Part model, mm, in its own coordinate system. Face numbers are marked on the shaded views. Round coordinates to 2 decimals unless told otherwise and drop trailing zeros. Loops run counter-clockwise (first coordinate to the right, second up) from the corner with the lowest first, then second, coordinate; pieces in that order, holes last. Notation, with made-up numbers: M 87.25,49 L 129.25,49 A31 cw 129.25,86 Z; hole C 89.5,5 d9. An arc over 180 degrees is marked long. Put each result on its own line as item: value. Start each with the question number.
1) Slice it at B-B on x = 7. Give the cut face in (y, z), then the cut area to 3 significant figures.
2) Probe line 1 along X through (y, z) = (30.1, 1.1); line 2 along Y through (x, z) = (30.1, 8); line 3 along X through (y, z) = (-28, 6). List the from-to ranges inside material, lowest first.
3) Slice it at C-C on x = -19. Give the cut face in (y, z), then the cut area to 3 significant figures.
4) Pull direction Y, two halves, no side cores. Call the marked faces 1 and 2: +Y half, -Y half, draft (parallel to the pull), parting line (faces both ways), or undercut.
5) Drop flat-ended pins along their axis: pin 1 Ø7 at (x, y) = (28.5, 28.5) entering from +Z; pin 2 Ø10 at (x, y) = (-26, -5) entering from +Z; pin 3 Ø2 at (x, z) = (7, 9.5) entering from -Y. Give the stop position or say it passes through.
6) Slice it at A-A on z = 9.5. State how many separate pieces and enclosed holes the cut face has, then the cut area to 3 significant figures.
```python
from build123d import *

# Parameters (mm, degrees)
SKETCH1_W            = 80.2
SKETCH1_H            = 80.2
BOSS_EXTRUDE1_DEPTH  = 4.5
M5_CLEARANCE_HOLE1_D = 5.3
FILLET1_R            = 10
SKETCH3_W            = 4
SKETCH3_H            = 18
BOSS_EXTRUDE2_DEPTH  = 10
CUT_EXTRUDE1_REACH   = 67.031
SKETCH5_R            = 2.4
CUT_EXTRUDE2_REACH   = 67.031
SKETCH6_R            = 1.75
FILLET2_R            = 2
FILLET3_R            = 4
BOSS_EXTRUDE3_START  = 6
SKETCH7_R            = 4.25
SKETCH7_R_2          = 2.65
BOSS_EXTRUDE3_DEPTH  = 6
FILLET5_R            = 1


with BuildPart() as part:
    # Sketch1 → Boss-Extrude1 (new body)
    with BuildSketch(Plane.XY):
        Rectangle(SKETCH1_W, SKETCH1_H)
    extrude(amount=BOSS_EXTRUDE1_DEPTH)

    # M5 Clearance Hole1 (through all)
    with Locations(Plane(origin=(30.1, 30.1, 0), x_dir=(-1, 0, 0), z_dir=(0, 0, -1))):
        with Locations((0, 0), (60.2, 0), (60.2, -60.2), (0, -60.2)):
            Hole(M5_CLEARANCE_HOLE1_D / 2)

    # Fillet1
    fillet1_edges = [part.edges().sort_by_distance(p)[0] for p in [
        (-40.1, -40.1, 2.25),
        (-40.1, 40.1, 2.25),
        (40.1, 40.1, 2.25),
        (40.1, -40.1, 2.25),
    ]]
    fillet(fillet1_edges, radius=FILLET1_R)

    # Sketch3 → Boss-Extrude2 (add)
    with BuildSketch(Plane.XY.offset(4.5)):
        with Locations((-7, 31.1)):
            Rectangle(SKETCH3_W, SKETCH3_H)
        with Locations((7, 31.1)):
            Rectangle(SKETCH3_W, SKETCH3_H)
    extrude(amount=BOSS_EXTRUDE2_DEPTH)

    # Sketch5 → Cut-Extrude1 (cut, up to next)
    with BuildSketch(Plane(origin=(9, 0, 0), x_dir=(0, 0, -1), z_dir=(1, 0, 0)), mode=Mode.PRIVATE) as cut_extrude1_sk1:
        with Locations(Location((-9.5, 36.1, 0), (0, 0, 90))):
            Circle(SKETCH5_R)
    cut_extrude1_tool1 = extrude(cut_extrude1_sk1.sketch, amount=-CUT_EXTRUDE1_REACH, mode=Mode.PRIVATE) & part.part
    # Sketch5 → Cut-Extrude1 (cut, up to next)
    with BuildSketch(Plane(origin=(9, 0, 0), x_dir=(0, 0, -1), z_dir=(1, 0, 0)), mode=Mode.PRIVATE) as cut_extrude1_sk2:
        with Locations(Location((-9.5, 26.1, 0), (0, 0, 90))):
            Circle(SKETCH5_R)
    cut_extrude1_tool2 = extrude(cut_extrude1_sk2.sketch, amount=-CUT_EXTRUDE1_REACH, mode=Mode.PRIVATE) & part.part
    add(cut_extrude1_tool1.solids().sort_by_distance((9, 36.1, 9.5))[0], mode=Mode.SUBTRACT)
    add(cut_extrude1_tool2.solids().sort_by_distance((9, 26.1, 9.5))[0], mode=Mode.SUBTRACT)

    # Sketch6 → Cut-Extrude2 (cut, up to next)
    with BuildSketch(Plane.ZY.offset(9), mode=Mode.PRIVATE) as cut_extrude2_sk1:
        with Locations((9.5, 36.1)):
            Circle(SKETCH6_R)
    cut_extrude2_tool1 = extrude(cut_extrude2_sk1.sketch, amount=-CUT_EXTRUDE2_REACH, mode=Mode.PRIVATE) & part.part
    # Sketch6 → Cut-Extrude2 (cut, up to next)
    with BuildSketch(Plane.ZY.offset(9), mode=Mode.PRIVATE) as cut_extrude2_sk2:
        with Locations((9.5, 26.1)):
            Circle(SKETCH6_R)
    cut_extrude2_tool2 = extrude(cut_extrude2_sk2.sketch, amount=-CUT_EXTRUDE2_REACH, mode=Mode.PRIVATE) & part.part
    add(cut_extrude2_tool1.solids().sort_by_distance((-9, 36.1, 9.5))[0], mode=Mode.SUBTRACT)
    add(cut_extrude2_tool2.solids().sort_by_distance((-9, 26.1, 9.5))[0], mode=Mode.SUBTRACT)

    # Fillet2
    fillet2_edges = [part.edges().sort_by_distance(p)[0] for p in [
        (-7, 22.1, 14.5),
        (-7, 40.1, 14.5),
        (7, 40.1, 14.5),
        (7, 22.1, 14.5),
    ]]
    fillet(fillet2_edges, radius=FILLET2_R)

    # Fillet3
    fillet3_edges = [part.edges().sort_by_distance(p)[0] for p in [
        (-7, 22.1, 4.5),
        (7, 22.1, 4.5),
    ]]
    fillet(fillet3_edges, radius=FILLET3_R)

    # Sketch7 → Boss-Extrude3 (add)
    # profile 1 of 4: a face of its own
    with BuildSketch(Plane.XY.offset(4.5).offset(BOSS_EXTRUDE3_START)):
        with Locations((-30.1, 30.1)):
            Circle(SKETCH7_R)
        with Locations(Location((-30.1, 30.1, 0), (0, 0, 180))):
            Circle(SKETCH7_R_2, mode=Mode.SUBTRACT)
    # profile 2 of 4: a face of its own
    with BuildSketch(Plane.XY.offset(4.5).offset(BOSS_EXTRUDE3_START)):
        with Locations((30.1, 30.1)):
            Circle(SKETCH7_R)
        with Locations(Location((30.1, 30.1, 0), (0, 0, 180))):
            Circle(SKETCH7_R_2, mode=Mode.SUBTRACT)
    # profile 3 of 4: a face of its own
    with BuildSketch(Plane.XY.offset(4.5).offset(BOSS_EXTRUDE3_START)):
        with Locations((30.1, -30.1)):
            Circle(SKETCH7_R)
        with Locations(Location((30.1, -30.1, 0), (0, 0, 180))):
            Circle(SKETCH7_R_2, mode=Mode.SUBTRACT)
    # profile 4 of 4: a face of its own
    with BuildSketch(Plane.XY.offset(4.5).offset(BOSS_EXTRUDE3_START)):
        with Locations((-30.1, -30.1)):
            Circle(SKETCH7_R)
        with Locations(Location((-30.1, -30.1, 0), (0, 0, 180))):
            Circle(SKETCH7_R_2, mode=Mode.SUBTRACT)
    extrude(amount=-BOSS_EXTRUDE3_DEPTH)

    # Fillet5
    fillet5_edges = [part.edges().sort_by_distance(p)[0] for p in [
        (-34.35, 30.1, 4.5),
        (25.85, 30.1, 4.5),
        (25.85, -30.1, 4.5),
        (-34.35, -30.1, 4.5),
    ]]
    fillet(fillet5_edges, radius=FILLET5_R)


solid = part.part
```
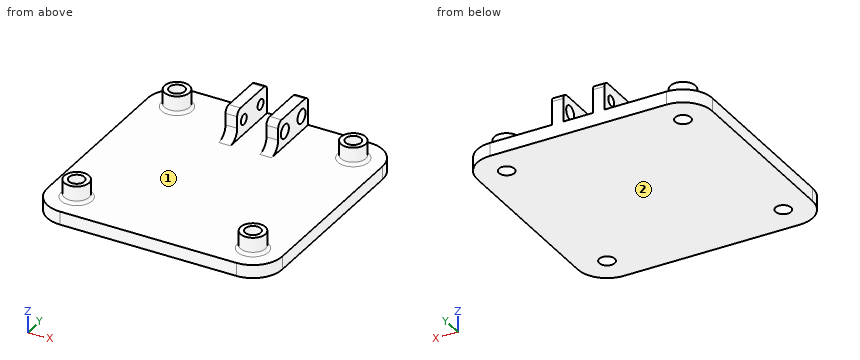
Recorded:
1. outline: M -40.1,0 L 40.1,0 L 40.1,12.5 A2 ccw 38.1,14.5 L 24.1,14.5 A2 ccw 22.1,12.5 L 22.1,8.5 A4 cw 18.1,4.5 L -40.1,4.5 Z; hole C 26.1,9.5 d4.8; hole C 36.1,9.5 d4.8
1. area: 506 mm2
2. line 1: x = -40.1 to -32.75, -27.45 to 27.45, 32.75 to 40.1
2. line 2: y = -34.35 to -32.75, -27.45 to -25.85, 25.85 to 27.45, 32.75 to 34.35
2. line 3: x = -33.79 to -31.72, -28.48 to -26.41, 26.41 to 28.48, 31.72 to 33.79
3. outline: M -40.1,0 L 40.1,0 L 40.1,4.5 L -40.1,4.5 Z
3. area: 361 mm2
4. face 1: undercut
4. face 2: draft
5. pin 1: stops at z = 10.5
5. pin 2: stops at z = 4.5
5. pin 3: stops at y = 22.1
6. separate pieces: 10
6. enclosed holes: 4
6. area: 216 mm2
